Could you check a few things on this model? Use its own coordinates, in mm. Face numbers are marked on the shaded views. A direction names the side the tool comes from. Coordinates: 2 decimals unless noted, no trailing zeros. Loops run counter-clockwise (first coordinate to the right, second up) from the corner with the lowest first, then second, coordinate; pieces in that order, holes last. Notation, with made-up numbers: (30, 62.25) -> (68, 62.25) arc R28 ccw to (68, 80.25) -> close; hole circle Ø11 at (60.5, 27.5). An arc over 180 degrees is marked (long way). One line per question, with ' | ' between items. Start each with the question number.
(1) Suppose I cut it at C-C (z = 6). Please give me the cut outline in (x, y).
(2) Suppose I cut it at A-A (x = 83). Please give me the cut outline in (y, z), plus the area to 3 significant figures.
(3) If I drill on line 1 along X through (y, z) = (69.5, 0.5); line 2 along Y through (x, z) = (2.5, 1.15); line 3 along Z through (x, y) = (29, 46.5), over which ranges is the centre line in solid material (lowest first)?
(4) Which directions (+Z, -Z, +X, -X, +Y, -Y) give clear straight access to the entire face, cutting with the end or side of a thin tool? Please do the marked faces 1, 2 and 3.
(5) Suppose I cut it at B-B (y = 26.5). Please give me the cut outline in (x, z), plus the area to 3 significant figures.
(6) I'm going to push flat-ended pins straight in: pin 1 Ø4 at (y, z) = (56, 4) entering from +X; pin 2 Ø2.5 at (x, y) = (103.5, 31) entering from +Z; pin 3 Ø7 at (x, z) = (89.5, 8) entering from +Y; pin 4 Ø1.6 at (x, y) = (2.5, 2.5) entering from +Z. Where does each tip first touch, or does it pass through?
```python
from build123d import *

# Parameters (mm, degrees)
MAIN_W                        = 100
MAIN_H                        = 72
MAIN_R                        = 1
MAIN_EXTRUSION_DEPTH          = 1.5
BOTTOM_HOLE_DEPTH             = 8.5
IDE_CONNECTOR_SKETCH_W        = 6
IDE_CONNECTOR_SKETCH_H        = 42
IDE_CONNECTOR_EXTRUSION_DEPTH = 8


with BuildPart() as part:
    # Main → Main-Extrusion (new body)
    with BuildSketch(Plane.XY):
        with Locations((50, 36)):
            Rectangle(MAIN_W, MAIN_H)
        with Locations((2.5, 69.5)):
            Circle(MAIN_R, mode=Mode.SUBTRACT)
        with Locations((2.5, 2.5)):
            Circle(MAIN_R, mode=Mode.SUBTRACT)
        with Locations((97.5, 69.5)):
            Circle(MAIN_R, mode=Mode.SUBTRACT)
        with Locations((97.5, 2.5)):
            Circle(MAIN_R, mode=Mode.SUBTRACT)
    extrude(amount=MAIN_EXTRUSION_DEPTH)

    # Bottom-Hole-Sketch → Bottom-Hole (add)
    with BuildSketch(Plane.XY.offset(1.5)):
        Polygon((0, 60), (69, 60), (69, 39), (100, 39), (100, 5), (69, 5), (0, 5), align=None)
    extrude(amount=BOTTOM_HOLE_DEPTH)

    # Ide-Connector-Sketch → Ide-Connector-Extrusion (add)
    with BuildSketch(Plane(origin=(100, 0, 0), x_dir=(0, 0, -1), z_dir=(1, 0, 0))):
        with Locations((-0.75, 31)):
            Rectangle(IDE_CONNECTOR_SKETCH_W, IDE_CONNECTOR_SKETCH_H)
    extrude(amount=IDE_CONNECTOR_EXTRUSION_DEPTH)


solid = part.part
```
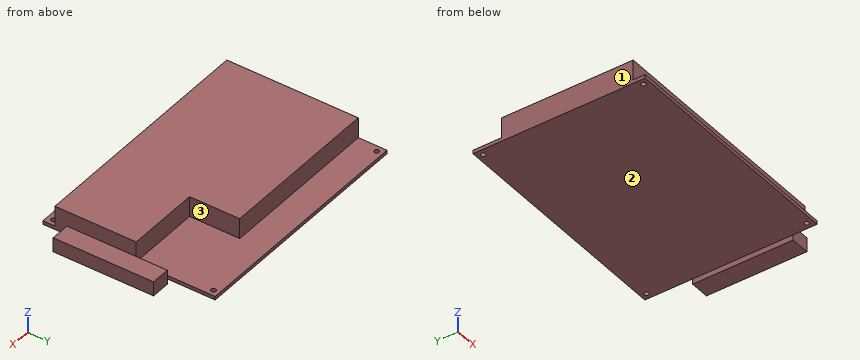
Checks:
1) outline: (0, 5) -> (100, 5) -> (100, 39) -> (69, 39) -> (69, 60) -> (0, 60) -> close
2) outline: (0, 0) -> (72, 0) -> (72, 1.5) -> (39, 1.5) -> (39, 10) -> (5, 10) -> (5, 1.5) -> (0, 1.5) -> close | area: 397 mm^2
3) line 1: x = 0 to 1.5, 3.5 to 96.5, 98.5 to 100 | line 2: y = 0 to 1.5, 3.5 to 68.5, 70.5 to 72 | line 3: z = 0 to 10
4) face 1: +Z, -Z, -X, +Y, -Y | face 2: -Z, -X, +Y, -Y | face 3: +Z, +Y
5) outline: (0, 0) -> (100, 0) -> (100, -2.25) -> (108, -2.25) -> (108, 3.75) -> (100, 3.75) -> (100, 10) -> (0, 10) -> close | area: 1,050 mm^2
6) pin 1: stops at x = 69 | pin 2: stops at z = 3.75 | pin 3: stops at y = 39 | pin 4: passes through
